Design review of the part built by this model. Coordinates are the model's own, in mm. A direction names the side the tool comes from. Round coordinates to 2 decimals unless told otherwise and drop trailing zeros. Loops run counter-clockwise (first coordinate to the right, second up) from the corner with the lowest first, then second, coordinate; pieces in that order, holes last. Notation, with made-up numbers: M -35.5,25.5 L 6.5,25.5 A19 cw 6.5,36.5 Z; hole C 7,25.25 d3. An arc over 180 degrees is marked long. Use a Markdown table: item, result.
from build123d import *

# Parameters (mm, degrees)
CROQUIS1_W              = 42.3
CROQUIS1_H              = 42.3
CROQUIS1_R              = 1.5
SALIENTE_EXTRUIR1_DEPTH = 6
REDONDEO1_R             = 5
CROQUIS2_R              = 11.2
CORTAR_EXTRUIR1_DEPTH   = 8
CROQUIS3_R              = 4.5
CORTAR_EXTRUIR2_DEPTH   = 10


with BuildPart() as part:
    # Croquis1 → Saliente-Extruir1 (new, symmetric)
    with BuildSketch(Plane.XY):
        Rectangle(CROQUIS1_W, CROQUIS1_H)
        with Locations((-15.5, 15.5)):
            Circle(CROQUIS1_R, mode=Mode.SUBTRACT)
        with Locations((-15.5, -15.5)):
            Circle(CROQUIS1_R, mode=Mode.SUBTRACT)
        with Locations(Location((15.5, -15.5, 0), (0, 0, 180))):
            Circle(CROQUIS1_R, mode=Mode.SUBTRACT)
        with Locations(Location((15.5, 15.5, 0), (0, 0, 180))):
            Circle(CROQUIS1_R, mode=Mode.SUBTRACT)
    extrude(amount=SALIENTE_EXTRUIR1_DEPTH, both=True)

    # Redondeo1
    redondeo1_edges = [part.edges().sort_by_distance(p)[0] for p in [
        (21.15, -21.15, 0),
        (-21.15, -21.15, 0),
        (-21.15, 21.15, 0),
        (21.15, 21.15, 0),
    ]]
    fillet(redondeo1_edges, radius=REDONDEO1_R)

    # Croquis2 → Cortar-Extruir1 (cut)
    with BuildSketch(Plane.XY.offset(6)):
        Circle(CROQUIS2_R)
    extrude(amount=-CORTAR_EXTRUIR1_DEPTH, mode=Mode.SUBTRACT)

    # Croquis3 → Cortar-Extruir2 (cut)
    with BuildSketch(Plane(origin=(0, 0, -6), x_dir=(-1, 0, 0), z_dir=(0, 0, -1))):
        Circle(CROQUIS3_R)
    extrude(amount=-CORTAR_EXTRUIR2_DEPTH, mode=Mode.SUBTRACT)


solid = part.part
1. Wall thickness on line 1 along Y through (x, z) = (0, -3.95); line 2 along X through (y, z) = (-16, 3); line 3 along Y through (x, z) = (5.5, 0.5): over which ranges is each line inside the solid? List them lowest first. Write a range as from..to.
Check values:
| item | result |
|---|---|
| line 1 | y = -21.15..-4.5, 4.5..21.15 |
| line 2 | x = -21.15..-16.91, -14.09..14.09, 16.91..21.15 |
| line 3 | y = -21.15..-9.76, 9.76..21.15 |
2. Machinability: for faces 1 (the face through (0.59, 4.46, -4.03)), 2 (the face through (-11.19, 0.49, 2.06)), which of the approach directions +Z, -Z, +X, -X, +Y, -Y give a long, thin tool a straight path to every point of the face, cutting with its end or side? Answer none if there is none.
Check values:
| item | result |
|---|---|
| face 1 | +Z, -Z |
| face 2 | +Z |
3. Take a section at C-C on z = -1.5. Give the boundary of the cut face in (x, y), and give its area (3 significant figures).
Check values:
| item | result |
|---|---|
| outline | M -21.15,-16.15 A5 ccw -16.15,-21.15 L 16.15,-21.15 A5 ccw 21.15,-16.15 L 21.15,16.15 A5 ccw 16.15,21.15 L -16.15,21.15 A5 ccw -21.15,16.15 Z; hole C -15.5,-15.5 d3; hole C -15.5,15.5 d3; hole C 0,0 d22.4; hole C 15.5,-15.5 d3; hole C 15.5,15.5 d3 |
| area | 1,350 mm² |
4. Take a section at A-A on x = 15.5. Give the boundary of the cut face in (y, z), and give its area (3 significant figures).
Check values:
| item | result |
|---|---|
| outline | M -21.15,-6 L -17,-6 L -17,6 L -21.15,6 Z; M -14,-6 L 14,-6 L 14,6 L -14,6 Z; M 17,-6 L 21.15,-6 L 21.15,6 L 17,6 Z |
| area | 436 mm² |
5. Take a section at D-D on x = 5. Give the boundary of the cut face in (y, z).
Check values:
| item | result |
|---|---|
| outline | M -21.15,-6 L 21.15,-6 L 21.15,6 L 10.02,6 L 10.02,-2 L -10.02,-2 L -10.02,6 L -21.15,6 Z |
6. The part is to be moulded in two halves that separate along X. For faces 3 (the face through (19.72, 19.65, -0.08)), 4 (the face through (0, -21.15, 0)), 5 (the face through (17, 15.43, -0.08)), say which applies: pulls with the +X half, pulls with the -X half, needs draft (parallel to the pull), parting line crosses it, or undercut.
Check values:
| item | result |
|---|---|
| face 3 | pulls with the +X half |
| face 4 | needs draft |
| face 5 | undercut |
